Here's how the part is built. I have some questions about the finished solid (model axes, mm). Give positions to 0.01 mm unless a question says otherwise; leave off trailing zeros. Write each loop counter-clockwise with the first axis right and the second up, starting at its lowest first coordinate (ties: lowest second). Pieces come first, ordered by that corner, then holes. Notation, with made-up numbers: (67, -33.5) -> (87, -33.5) arc R7 cw to (87, -27.5) -> close; hole circle Ø9 at (30.25, 54.25). An arc over 180 degrees is marked (long way). Return JSON: item names as keys, results as strings.
from build123d import *

# Parameters (mm, degrees)
SKETCH1_W           = 880
SKETCH1_H           = 580
BOSS_EXTRUDE1_DEPTH = 60
SKETCH2_R           = 30
CUT_EXTRUDE1_DEPTH  = 260
SKETCH4_R           = 4
CUT_EXTRUDE3_DEPTH  = 260


with BuildPart() as part:
    # Sketch1 → Boss-Extrude1 (new body)
    with BuildSketch(Plane(origin=(0, 0, 0), x_dir=(1, 0, 0), z_dir=(0, 1, 0))):
        Rectangle(SKETCH1_W, SKETCH1_H)
    extrude(amount=BOSS_EXTRUDE1_DEPTH)

    # Sketch2 → Cut-Extrude1 (cut)
    with BuildSketch(Plane(origin=(0, 60, 0), x_dir=(1, 0, 0), z_dir=(0, 1, 0))):
        with Locations(Location((-340, 200, 0), (0, 0, 270))):
            Circle(SKETCH2_R)
        with Locations(Location((340, 200, 0), (0, 0, 270))):
            Circle(SKETCH2_R)
        with Locations(Location((340, -200, 0), (0, 0, 270))):
            Circle(SKETCH2_R)
        with Locations(Location((-340, -200, 0), (0, 0, 270))):
            Circle(SKETCH2_R)
    extrude(amount=-CUT_EXTRUDE1_DEPTH, mode=Mode.SUBTRACT)

    # Sketch4 → Cut-Extrude3 (cut)
    with BuildSketch(Plane(origin=(0, 60, 0), x_dir=(1, 0, 0), z_dir=(0, 1, 0))):
        with Locations(Location((-129.655068581, 29.344931419, 0), (0, 0, 270))):
            Circle(SKETCH4_R)
        with Locations(Location((-129.655068581, -29.344931419, 0), (0, 0, 270))):
            Circle(SKETCH4_R)
        with Locations(Location((-188.344931419, -29.344931419, 0), (0, 0, 270))):
            Circle(SKETCH4_R)
        with Locations(Location((-188.344931419, 29.344931419, 0), (0, 0, 270))):
            Circle(SKETCH4_R)
        with Locations(Location((188.344931419, 29.344931419, 0), (0, 0, 270))):
            Circle(SKETCH4_R)
        with Locations(Location((188.344931419, -29.344931419, 0), (0, 0, 270))):
            Circle(SKETCH4_R)
        with Locations(Location((129.655068581, -29.344931419, 0), (0, 0, 270))):
            Circle(SKETCH4_R)
        with Locations(Location((129.655068581, 29.344931419, 0), (0, 0, 270))):
            Circle(SKETCH4_R)
    extrude(amount=-CUT_EXTRUDE3_DEPTH, mode=Mode.SUBTRACT)


solid = part.part
1. If I drill on line 1 (X direction, y = 25, z = -28), over which ranges is the centre line in solid material (lowest first)? Write a range as [from, to].
Taken from the geometry:
{"line 1": "x = [-440, -192.11], [-184.58, -133.42], [-125.89, 125.89], [133.42, 184.58], [192.11, 440]"}
2. If we mould it in two halves opening along Z, with no side actions, what happens to faces 1 (the face through (-6, 0, -4)), 2 (the face through (-366.615, 30.42, 213.843)), 3 (the face through (-6, 30, 290))? For each: released by +Z, released by -Z, zero draft, split by the parting line, or undercut.
Taken from the geometry:
{"face 1": "zero draft", "face 2": "undercut", "face 3": "released by +Z"}
3. Suppose I cut it at A-A, the plane z = -200. List the corners of the cut face in (x, y) for me, and give its area (3 significant figures).
Taken from the geometry:
{"outline": "(-440, 0) -> (-370, 0) -> (-370, 60) -> (-440, 60) -> close; (-310, 0) -> (310, 0) -> (310, 60) -> (-310, 60) -> close; (370, 0) -> (440, 0) -> (440, 60) -> (370, 60) -> close", "area": "45,600 mm²"}
4. Suppose I cut it at B-B, the plane x = -340. List the corners of the cut face in (y, z) for me, and give its area (3 significant figures).
Taken from the geometry:
{"outline": "(0, -290) -> (60, -290) -> (60, -230) -> (0, -230) -> close; (0, -170) -> (60, -170) -> (60, 170) -> (0, 170) -> close; (0, 230) -> (60, 230) -> (60, 290) -> (0, 290) -> close", "area": "27,600 mm²"}
5. Suppose I cut it at C-C, the plane y = 31. Count the separate pieces of the cut face and the enclosed holes in it, and give its area (3 significant figures).
Taken from the geometry:
{"separate pieces": "1", "enclosed holes": "12", "area": "499,000 mm²"}
6. For pin 1 Ø5 at (x, z) = (188.34, -29.34) entering from +Y, with a flat end and sliding along its axis, tell me the tip position at first contact or that it passes through.
Taken from the geometry:
{"pin 1": "passes through"}
